```python
from build123d import *

# Parameters (mm, degrees)
F0_R     = 76.2
F1_DEPTH = 12.7
F2_R     = 12.2642048969
F3_R     = 11.0377844072


# Not quite as in the source:
# - ends of sketch curves that miss each other by under 0.0002 mm in the source are joined
# - a feature names something its author has since deleted; it is built from what else it names


with BuildPart() as f1:
    # F0 (on Top) → F1 (new body, symmetric)
    with BuildSketch(Plane.XY):
        Circle(F0_R)
        with BuildLine():
            ThreePointArc((49.1868885365, 12.6999998465), (50.3951085804, 6.4010179795), (50.8, 0))
            ThreePointArc((50.8, 0), (50.3951085804, -6.4010179795), (49.1868885365, -12.6999998465))
            ThreePointArc((49.1868885365, -12.6999998465), (35.9210245403, -35.9210244282), (12.7, -49.1868884968))
            ThreePointArc((12.7, -49.1868884968), (6.4010180581, -50.3951085704), (0, -50.8))
            ThreePointArc((0, -50.8), (-6.4010180581, -50.3951085704), (-12.7, -49.1868884968))
            ThreePointArc((-12.7, -49.1868884968), (-35.9210245403, -35.9210244282), (-49.1868885365, -12.6999998465))
            ThreePointArc((-49.1868885365, -12.6999998465), (-50.3951085804, -6.4010179795), (-50.8, 0))
            ThreePointArc((-50.8, 0), (-50.3951085704, 6.4010180581), (-49.1868884968, 12.7))
            ThreePointArc((-49.1868884968, 12.7), (-35.9210244282, 35.9210245403), (-12.6999998465, 49.1868885365))
            ThreePointArc((-12.6999998465, 49.1868885365), (-6.4010179795, 50.3951085804), (0, 50.8))
            ThreePointArc((0, 50.8), (6.4010179795, 50.3951085804), (12.6999998465, 49.1868885365))
            ThreePointArc((12.6999998465, 49.1868885365), (35.9210244843, 35.9210244843), (49.1868885365, 12.6999998465))
        make_face(mode=Mode.SUBTRACT)
        with BuildLine():
            ThreePointArc((12.7, -49.1868884968), (35.9210245403, -35.9210244282), (49.1868885365, -12.6999998465))
            Line((49.1868885365, -12.6999998465), (14.1990317944, -12.6999998465))
            Line((14.1990317944, -12.6999998465), (12.7, -12.6999998465))
            Line((12.7, -12.6999998465), (12.7, -14.1990316571))
            Line((12.7, -14.1990316571), (12.7, -49.1868884968))
        make_face()
        with BuildLine():
            ThreePointArc((-49.1868885365, -12.6999998465), (-35.9210245403, -35.9210244282), (-12.7, -49.1868884968))
            Line((-12.7, -49.1868884968), (-12.7, -14.1990316571))
            Line((-12.7, -14.1990316571), (-12.7, -12.6999998465))
            Line((-12.7, -12.6999998465), (-14.1990317944, -12.6999998465))
            Line((-14.1990317944, -12.6999998465), (-49.1868885365, -12.6999998465))
        make_face()
        with BuildLine():
            Line((-12.6999998465, 14.1990317944), (-12.6999998465, 49.1868885365))
            ThreePointArc((-12.6999998465, 49.1868885365), (-35.9210244282, 35.9210245403), (-49.1868884968, 12.7))
            Line((-49.1868884968, 12.7), (-14.1990316571, 12.7))
            Line((-14.1990316571, 12.7), (-12.6999998465, 12.7))
            Line((-12.6999998465, 12.7), (-12.6999998465, 14.1990317944))
        make_face()
        with BuildLine():
            Line((14.1990317944, 12.6999998465), (49.1868885365, 12.6999998465))
            ThreePointArc((49.1868885365, 12.6999998465), (35.9210244843, 35.9210244843), (12.6999998465, 49.1868885365))
            Line((12.6999998465, 49.1868885365), (12.6999998465, 14.1990317944))
            Line((12.6999998465, 14.1990317944), (12.6999998465, 12.6999998465))
            Line((12.6999998465, 12.6999998465), (14.1990317944, 12.6999998465))
        make_face()
        Polygon((12.7, -12.6999998465), (12.7, 0), (12.6999998465, 12.6999998465), (0, 12.6999998465), (-12.6999998465, 12.7), (-12.7, 0), (-12.7, -12.6999998465), (0, -12.6999998465), align=None)
        with BuildLine():
            Line((-12.7, 0), (-12.6999998465, 12.7))
            Line((-12.6999998465, 12.7), (-14.1990316571, 12.7))
            ThreePointArc((-14.1990316571, 12.7), (-17.7959834382, 6.7974608102), (-19.05, 0))
            Line((-19.05, 0), (-12.7, 0))
        make_face()
        with BuildLine():
            ThreePointArc((14.1990317944, -12.6999998465), (17.795983475, -6.797460714), (19.05, 0))
            Line((19.05, 0), (12.7, 0))
            Line((12.7, 0), (12.7, -12.6999998465))
            Line((12.7, -12.6999998465), (14.1990317944, -12.6999998465))
        make_face()
        with BuildLine():
            Line((12.7, 0), (19.05, 0))
            ThreePointArc((19.05, 0), (17.795983475, 6.797460714), (14.1990317944, 12.6999998465))
            Line((14.1990317944, 12.6999998465), (12.6999998465, 12.6999998465))
            Line((12.6999998465, 12.6999998465), (12.7, 0))
        make_face()
        with BuildLine():
            ThreePointArc((0, -19.05), (6.7974608102, -17.7959834382), (12.7, -14.1990316571))
            Line((12.7, -14.1990316571), (12.7, -12.6999998465))
            Line((12.7, -12.6999998465), (0, -12.6999998465))
            Line((0, -12.6999998465), (0, -19.05))
        make_face()
        with BuildLine():
            ThreePointArc((-12.7, -14.1990316571), (-6.7974608102, -17.7959834382), (0, -19.05))
            Line((0, -19.05), (0, -12.6999998465))
            Line((0, -12.6999998465), (-12.7, -12.6999998465))
            Line((-12.7, -12.6999998465), (-12.7, -14.1990316571))
        make_face()
        with BuildLine():
            Line((-14.1990317944, -12.6999998465), (-12.7, -12.6999998465))
            Line((-12.7, -12.6999998465), (-12.7, 0))
            Line((-12.7, 0), (-19.05, 0))
            ThreePointArc((-19.05, 0), (-17.795983475, -6.797460714), (-14.1990317944, -12.6999998465))
        make_face()
        with BuildLine():
            Line((0, 12.6999998465), (0, 19.05))
            ThreePointArc((0, 19.05), (-6.797460714, 17.795983475), (-12.6999998465, 14.1990317944))
            Line((-12.6999998465, 14.1990317944), (-12.6999998465, 12.7))
            Line((-12.6999998465, 12.7), (0, 12.6999998465))
        make_face()
        with BuildLine():
            Line((12.6999998465, 12.6999998465), (12.6999998465, 14.1990317944))
            ThreePointArc((12.6999998465, 14.1990317944), (6.797460714, 17.795983475), (0, 19.05))
            Line((0, 19.05), (0, 12.6999998465))
            Line((0, 12.6999998465), (12.6999998465, 12.6999998465))
        make_face()
    extrude(amount=F1_DEPTH, both=True)

    # F2
    f2_edges = [f1.edges().sort_by_distance(p)[0] for p in [
        (-76.2, 0, 12.7),
    ]]
    fillet(f2_edges, radius=F2_R)

    # F3
    f3_edges = [f1.edges().sort_by_distance(p)[0] for p in [
        (-76.2, 0, -12.7),
    ]]
    fillet(f3_edges, radius=F3_R)


solid = f1.part
```
Could you check a few things on this model? Use its own coordinates, in mm. A direction names the side the tool comes from. Round coordinates to 2 decimals unless told otherwise and drop trailing zeros. Loops run counter-clockwise (first coordinate to the right, second up) from the corner with the lowest first, then second, coordinate; pieces in that order, holes last.
Q1. I want a section at D-D (z = -8.25). Write out the boundary of the cut face in (x, y).
Q2. Thinking about a two-plate mould opening in Y: for faces 3 (the cylindrical face through (-60.47, -46.367, -0.599)), 4 (the flat face through (-1, 1, 12.7)), 5 (the cylindrical face through (-50.8, -0.2, 0.2)), which applies, pulls with the +Y half, pulls with the -Y half, needs draft (parallel to the pull), parting line crosses it, or undercut?
Q3. I want a section at C-C (z = 9.25). Write out the boundary of the cut face in (x, y), and give its area (3 significant figures).
Q4. For P1, Ø8, axis at x = 24, z = -1.5, coming from the -Y side; P2, Ø7.5, axis at y = -35, z = -5, coming from the -X side; P3, Ø12, axis at x = -46.5, z = -2, coming from the -Y side, each with a flat end and sliding along its axis, tell me the tip position at first contact or that it passes through.
Q5. I want a section at A-A (y = 0). Write out the boundary of the cut face in (x, z).
Q6. Please list where these lines run through material, in increasing order: L1, parallel to Y at x = -16.5, z = 0; L2, parallel to Y at x = 9.5, z = -1.25; L3, parallel to X at y = 5, z = 2.75.
Q7. On a 3-axis mill with a long thin cutter (end or side, diameter ignored), from which of +Z, -Z, +X, -X, +Y, -Y can I reach the whole of each face in a straight line? I mean faces 1 (the flat face through (-1, 1, -12.7)), 2 (the cylindrical face through (-0.2, 50.8, 0.2)). Say none if no direction works.
Answer below:
1. outline: circle Ø148.04 at (0, 0); hole (-49.19, -12.7) - (-14.2, -12.7) arc R19.05 cw to (-14.2, 12.7) - (-49.19, 12.7) arc R50.8 ccw to start; hole (-12.7, -49.19) arc R50.8 ccw to (12.7, -49.19) - (12.7, -14.2) arc R19.05 cw to (-12.7, -14.2) - close; hole (-12.7, 14.2) arc R19.05 cw to (12.7, 14.2) - (12.7, 49.19) arc R50.8 ccw to (-12.7, 49.19) - close; hole (14.2, -12.7) - (49.19, -12.7) arc R50.8 ccw to (49.19, 12.7) - (14.2, 12.7) arc R19.05 cw to start
2. face 3: parting line crosses it
2. face 4: needs draft
2. face 5: undercut
3. outline: circle Ø144.93 at (0, 0); hole (-49.19, -12.7) - (-14.2, -12.7) arc R19.05 cw to (-14.2, 12.7) - (-49.19, 12.7) arc R50.8 ccw to start; hole (-12.7, -49.19) arc R50.8 ccw to (12.7, -49.19) - (12.7, -14.2) arc R19.05 cw to (-12.7, -14.2) - close; hole (-12.7, 14.2) arc R19.05 cw to (12.7, 14.2) - (12.7, 49.19) arc R50.8 ccw to (-12.7, 49.19) - close; hole (14.2, -12.7) - (49.19, -12.7) arc R50.8 ccw to (49.19, 12.7) - (14.2, 12.7) arc R19.05 cw to start
3. area: 13,200 mm2
4. P1: stops at y = -73.53
4. P2: stops at x = -69.19
4. P3: stops at y = -64.54
5. outline: (-76.2, -1.66) arc R11.04 ccw to (-65.16, -12.7) - (-50.8, -12.7) - (-50.8, 12.7) - (-63.94, 12.7) arc R12.26 ccw to (-76.2, 0.44) - close; (-19.05, -12.7) - (19.05, -12.7) - (19.05, 12.7) - (-19.05, 12.7) - close; (50.8, -12.7) - (65.16, -12.7) arc R11.04 ccw to (76.2, -1.66) - (76.2, 0.44) arc R12.26 ccw to (63.94, 12.7) - (50.8, 12.7) - close
6. L1: y = -74.39 to -12.7, -9.52 to 9.52, 12.7 to 74.39
6. L2: y = -75.61 to -49.9, -16.51 to 16.51, 49.9 to 75.61
6. L3: x = -75.81 to -50.55, -18.38 to 18.38, 50.55 to 75.81
7. face 1: -Z, +X, -X, +Y, -Y
7. face 2: +Z, -Z
